The model under review builds one solid part; all positions refer to its coordinate system, in mm. Face numbers are marked on the shaded views. A direction names the side the tool comes from. Coordinates: 2 decimals unless noted, no trailing zeros. Order: outer loops, then holes, each group sorted by start corner. A loop starts at its lowest first (then second) coordinate and runs counter-clockwise, first axis right, second up. Notation, with made-up numbers: (45.5, -30) -> (92.5, -30) arc R18 cw to (92.5, 3) -> close; hole circle Ø1 at (-26.5, 32.5). An arc over 180 degrees is marked (long way). Answer as CSV lines item,"result". Start each with the question number.
from build123d import *

# Parameters (mm, degrees)
POCKET_DEPTH       = 56.871497
POLARPATTERN_COUNT = 36


with BuildPart() as part:
    # Sketch → Revolution (revolve)
    with BuildSketch(Plane.YZ):
        Polygon((0, 0), (0, 1.195), (0.176092, 1.5), (6, 1.5), (6, 3), (11, 3), (11, 5.5), (11.5, 6), (13, 6), (13.5, 5.5), (13.5, 0), align=None)
    revolve(axis=Axis((0, 0, 0), (0, 1, 0)))

    # Sketch001 → Pocket (cut, through all)
    with BuildSketch(Plane.ZX.offset(13.5)):
        Polygon((-0.5, 6.05), (0, 5.55), (0.5, 6.05), align=None)
    pocket = extrude(amount=-POCKET_DEPTH, mode=Mode.SUBTRACT)

    # PolarPattern: Pocket ×36 about axis
    polarpattern_axis = Axis((0, 13.5, 0), (0, 1, 0))
    for i in range(1, POLARPATTERN_COUNT):
        add(pocket.rotate(polarpattern_axis, i * 360 / POLARPATTERN_COUNT), mode=Mode.SUBTRACT)


solid = part.part
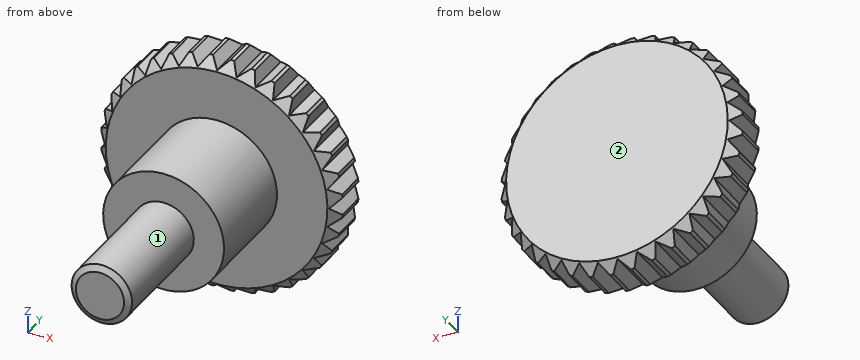
1) Consider section B-B (y = 1.5). Give the boundary of the cut face in (x, z), plus the area to 3 significant figures.
2) Consider section A-A (y = 7.5). Give the boundary of the cut face in (x, z), plus the area to 3 significant figures.
3) Wall thickness on L1, parallel to Y at x = 3.5, z = 3; L2, parallel to X at y = 12.5, z = 3; L3, parallel to Z at x = -2.5, y = 9: over which ranges is each line inside the solid? List them lowest first. Write a range as [from, to].
4) Tool access review of the marked faces 1 and 2: name each direction out of +Z, -Z, +X, -X, +Y, -Y from which nothing blocks a thin tool from reaching the whole face with its end or side.
5) Insertion check: pin 1 Ø1.5 at (y, z) = (5, 0) entering from -X; pin 2 Ø3 at (x, y) = (1, 1.5) entering from +Z; pin 3 Ø1.5 at (x, z) = (4.5, 1) entering from -Y. Each pin has a flat end and moves straight along its axis. Give the tip position at first contact, or say it passes through.
Result:
1,outline,"circle Ø3 at (0, 0)"
1,area,"7.07 mm2"
2,outline,"circle Ø6 at (0, 0)"
2,area,"28.3 mm2"
3,L1,"[11, 13.5]"
3,L2,"[-4.87, 4.87]"
3,L3,"[-1.66, 1.66]"
4,face 1,"-Y"
4,face 2,"+Z, -Z, +X, -X, +Y"
5,pin 1,"x = -1.5"
5,pin 2,"z = 1.5"
5,pin 3,"y = 11"
